Verification items for the finished model (mm, model axes). A direction names the side the tool comes from. Give positions to 0.01 mm unless a question says otherwise; leave off trailing zeros. Write each loop counter-clockwise with the first axis right and the second up, starting at its lowest first coordinate (ties: lowest second). Pieces come first, ordered by that corner, then holes. Notation, with made-up numbers: (-36, 15) -> (0, 15) arc R21 ccw to (0, 42) -> close; hole circle Ø10 at (48, 69.5). An arc over 180 degrees is marked (long way). Write item = value, one per line.
from build123d import *

# Parameters (mm, degrees)
SKETCH2_W           = 95.25
SKETCH2_H           = 25.4
SKETCH2_R           = 6.35
EXTRUDE1_DEPTH      = 3.175
EXTRUDE1_2_DEPTH    = 3.175
SKETCH3_W           = 38.1
SKETCH3_H           = 115.8875
EXTRUDE2_DEPTH      = 25.4
SKETCH4_W           = 33.02
SKETCH4_H           = 20.32
EXTRUDE3_DEPTH      = 38.1
SKETCH5_W           = 133.35
SKETCH5_H           = 20.32
EXTRUDE4_DEPTH      = 3.175
CUT_EXTRUDE1_DEPTH  = 158.1625
EXTRUDE5_DEPTH      = 3.175
SKETCH9_R           = 6.35
EXTRUDE6_DEPTH      = 3.175
SKETCH10_W          = 254
SKETCH10_H          = 115.8875
EXTRUDE7_DEPTH      = 6.35
SKETCH11_R          = 6.35
CUT_EXTRUDE2_DEPTH  = 7.35
SKETCH12_R          = 6.35
CUT_EXTRUDE3_DEPTH  = 35.925
LPATTERN1_COUNT     = 3
LPATTERN1_PITCH     = 19.05
LPATTERN1_COL_COUNT = 3
LPATTERN1_COL_PITCH = 19.05


with BuildPart() as part:
    # Sketch2 → Extrude1 (new body)
    with BuildSketch(Plane.XY):
        with Locations((0, -45.24375)):
            Rectangle(SKETCH2_W, SKETCH2_H)
        with Locations((-33.3375, -45.24375)):
            Circle(SKETCH2_R, mode=Mode.SUBTRACT)
        with Locations((33.3375, -45.24375)):
            Circle(SKETCH2_R, mode=Mode.SUBTRACT)
    extrude(amount=EXTRUDE1_DEPTH)



with BuildPart() as body_2:
    # Sketch2 → Extrude1 2 (new body)
    with BuildSketch(Plane.XY):
        with Locations((0, 45.24375)):
            Rectangle(SKETCH2_W, SKETCH2_H)
        with Locations((33.3375, 45.24375)):
            Circle(SKETCH2_R, mode=Mode.SUBTRACT)
        with Locations((-33.3375, 45.24375)):
            Circle(SKETCH2_R, mode=Mode.SUBTRACT)
    extrude(amount=EXTRUDE1_2_DEPTH)


with BuildPart() as part_1:
    add(part.part)

    add(body_2.part)  # Extrude2 merges body 2
    # Sketch3 → Extrude2 (add)
    with BuildSketch(Plane.XY.offset(3.175)):
        Rectangle(SKETCH3_W, SKETCH3_H)
    extrude(amount=EXTRUDE2_DEPTH)

    # Sketch4 → Extrude3 (add)
    with BuildSketch(Plane(origin=(0, 57.94375, 0), x_dir=(1, 0, 0), z_dir=(0, 1, 0))):
        with Locations((0, -15.875)):
            Rectangle(SKETCH4_W, SKETCH4_H)
    extrude(amount=EXTRUDE3_DEPTH)

    # Sketch5 → Extrude4 (add)
    with BuildSketch(Plane(origin=(0, 96.04375, 0), x_dir=(1, 0, 0), z_dir=(0, 1, 0))):
        with Locations((0, -15.875)):
            Rectangle(SKETCH5_W, SKETCH5_H)
    extrude(amount=EXTRUDE4_DEPTH)

    # Sketch6 → Cut-Extrude1 (cut, through all)
    with BuildSketch(Plane(origin=(0, 99.21875, 0), x_dir=(1, 0, 0), z_dir=(0, 1, 0))):
        with BuildLine():
            Line((54.76875, -20.6375), (37.30625, -20.6375))
            ThreePointArc((37.30625, -20.6375), (32.54375, -15.875), (37.30625, -11.1125))
            Line((37.30625, -11.1125), (54.76875, -11.1125))
            ThreePointArc((54.76875, -11.1125), (59.53125, -15.875), (54.76875, -20.6375))
        make_face()
        with BuildLine():
            Line((-54.76875, -11.1125), (-37.30625, -11.1125))
            ThreePointArc((-37.30625, -11.1125), (-32.54375, -15.875), (-37.30625, -20.6375))
            Line((-37.30625, -20.6375), (-54.76875, -20.6375))
            ThreePointArc((-54.76875, -20.6375), (-59.53125, -15.875), (-54.76875, -11.1125))
        make_face()
    extrude(amount=-CUT_EXTRUDE1_DEPTH, mode=Mode.SUBTRACT)

    # Sketch8 → Extrude5 (add)
    with BuildSketch(Plane.XZ.offset(57.94375)):
        Polygon((12.065, 6.965730998), (12.065, 20.897192993), (0, 27.862923991), (-12.065, 20.897192993), (-12.065, 6.965730998), (0, 0), align=None)
    extrude(amount=EXTRUDE5_DEPTH)

    # Sketch9 → Extrude6 (add)
    with BuildSketch(Plane.XZ.offset(61.11875)):
        with Locations((0, 13.931461996)):
            Circle(SKETCH9_R)
    extrude(amount=EXTRUDE6_DEPTH)

    # Sketch10 → Extrude7 (add)
    with BuildSketch(Plane(origin=(0, 0, 0), x_dir=(-1, 0, 0), z_dir=(0, 0, -1))):
        Rectangle(SKETCH10_W, SKETCH10_H)
    extrude(amount=EXTRUDE7_DEPTH)

    # Sketch11 → Cut-Extrude2 (cut, through all)
    with BuildSketch(Plane.XY):
        with Locations((33.3375, -45.24375)):
            Circle(SKETCH11_R)
        with Locations((-33.3375, -45.24375)):
            Circle(SKETCH11_R)
        with Locations((-33.3375, 45.24375)):
            Circle(SKETCH11_R)
        with Locations((33.3375, 45.24375)):
            Circle(SKETCH11_R)
    extrude(amount=-CUT_EXTRUDE2_DEPTH, mode=Mode.SUBTRACT)

    # Sketch12 → Cut-Extrude3 (cut, through all)
    with BuildSketch(Plane(origin=(0, 0, -6.35), x_dir=(-1, 0, 0), z_dir=(0, 0, -1))):
        with Locations((-111.125, 0)):
            Circle(SKETCH12_R)
        with Locations((111.125, 0)):
            Circle(SKETCH12_R)
    cut_extrude3 = extrude(amount=-CUT_EXTRUDE3_DEPTH, mode=Mode.SUBTRACT)

    # LPattern1: Cut-Extrude3 ×3
    with Locations(*[(0, i * LPATTERN1_PITCH, 0) for i in range(1, LPATTERN1_COUNT)]):
        add(cut_extrude3, mode=Mode.SUBTRACT)

    # LPattern1 col: Cut-Extrude3 ×3
    with Locations(*[(0, -i * LPATTERN1_COL_PITCH, 0) for i in range(1, LPATTERN1_COL_COUNT)]):
        add(cut_extrude3, mode=Mode.SUBTRACT)


solid = part_1.part
Item 1: Material ranges on line 1 (X direction, y = 19, z = -3); line 2 (Y direction, x = -25, z = 1); line 3 (Z direction, x = 14, y = 22) (3 decimals), recorded low to high.
Response values:
line_1 = -127 to -117.47, -104.78 to 104.78, 117.47 to 127
line_2 = -57.94 to -32.54, 32.54 to 57.94
line_3 = -6.35 to 0, 3.175 to 28.575
Item 2: Sectioned sample at A-A on y = 19.05. Record the cut outline in (x, z) (3 decimals).
Response values:
outline = (-127, -6.35) -> (-117.475, -6.35) -> (-117.475, 0) -> (-127, 0) -> close; (-104.775, -6.35) -> (104.775, -6.35) -> (104.775, 0) -> (-104.775, 0) -> close; (-19.05, 3.175) -> (19.05, 3.175) -> (19.05, 28.575) -> (-19.05, 28.575) -> close; (117.475, -6.35) -> (127, -6.35) -> (127, 0) -> (117.475, 0) -> close
Item 3: Set-up check for faces 4 (the cylindrical face through (32.545, 97.653, 15.98)), 5 (the flat face through (-16.51, 77, 16)), 6 (the flat face through (26.8, 45.4, 3.175)), 7 (the flat face through (6.12, -59.51, 24.33)): record each of +Z, -Z, +X, -X, +Y, -Y from which the full face is reachable in a straight line by a thin tool's end or side.
Response values:
face_4 = +Y, -Y
face_5 = +Z, -Z, -X
face_6 = +Z, +X, +Y, -Y
face_7 = +Z, +X, -Y
Item 4: Go/stop test with flat-tipped pins: P1, Ø1, axis at y = -48.5, z = 1.5, coming from the -X side (3 decimals); P2, Ø16.5, axis at y = 76, z = 12.5, coming from the -X side; P3, Ø12.5, axis at x = 39, y = 51.5, coming from the +Z side (3 decimals); P4, Ø8, axis at y = -32.5, z = 2.5, coming from the -X side. Record where each tip stops, or that it passes through.
Response values:
P1 = -47.625
P2 = -16.51
P3 = 3.175
P4 = -127
Item 5: Sectioned sample at B-B on x = -108.5. Record the cut outline in (y, z).
Response values:
outline = (-57.94, -6.35) -> (-43.88, -6.35) -> (-43.88, 0) -> (-57.94, 0) -> close; (-32.32, -6.35) -> (-24.83, -6.35) -> (-24.83, 0) -> (-32.32, 0) -> close; (-13.27, -6.35) -> (-5.78, -6.35) -> (-5.78, 0) -> (-13.27, 0) -> close; (5.78, -6.35) -> (13.27, -6.35) -> (13.27, 0) -> (5.78, 0) -> close; (24.83, -6.35) -> (32.32, -6.35) -> (32.32, 0) -> (24.83, 0) -> close; (43.88, -6.35) -> (57.94, -6.35) -> (57.94, 0) -> (43.88, 0) -> close
Item 6: Mould release check, pull along Y, two halves, no side actions. Record for faces 1 (the flat face through (-1, 99.219, 16)), 2 (the cylindrical face through (108.19, 32.47, -3.22)), 3 (the flat face through (-6.117, -59.509, 3.532)): +Y half, -Y half, draft (parallel to the pull), parting line (faces both ways), or undercut.
Response values:
face_1 = +Y half
face_2 = undercut
face_3 = draft
Item 7: Sectioned sample at C-C on x = 81. Record the cut outline in (y, z), then the cut area to 3 significant figures.
Response values:
outline = (-57.94, -6.35) -> (57.94, -6.35) -> (57.94, 0) -> (-57.94, 0) -> close
area = 736 mm^2
